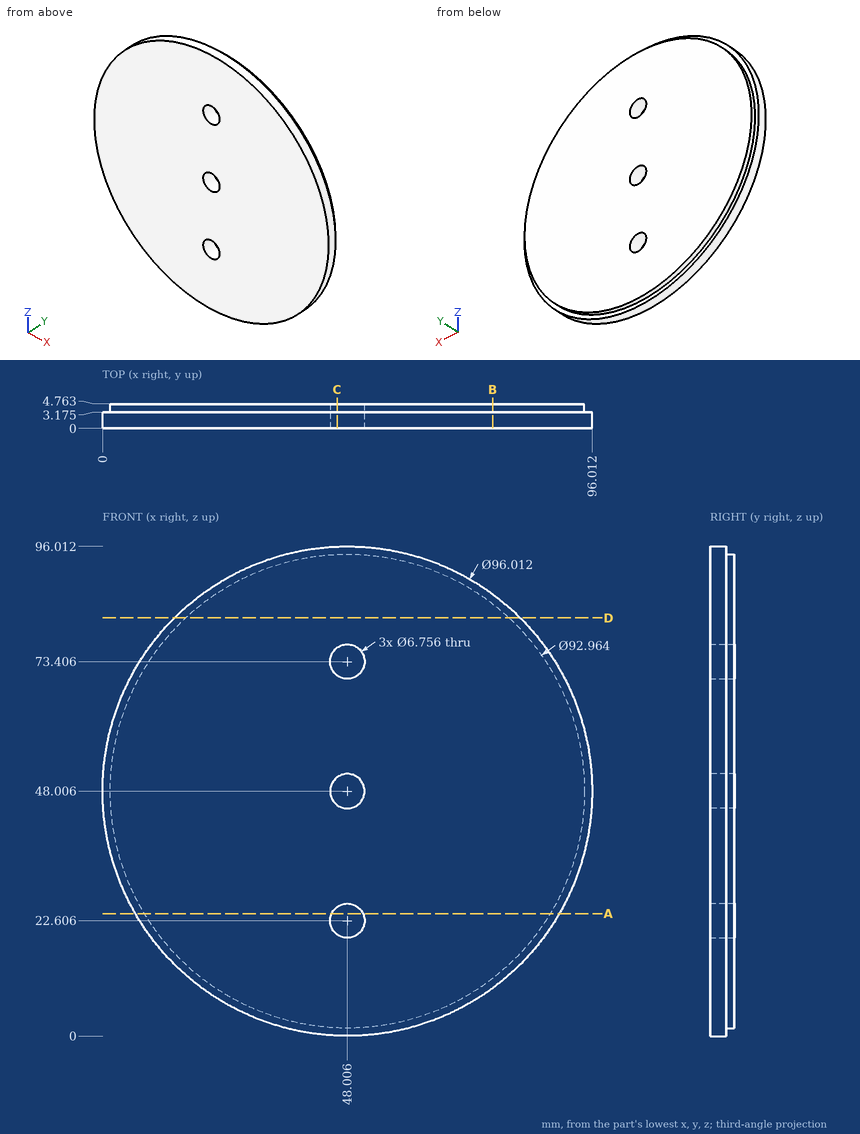
Geometry: see drawing. Coordinates: mm, zero at the bounding-box minimum. Round coordinates to 2 decimals unless told otherwise and drop trailing zeros. Loops run counter-clockwise (first coordinate to the right, second up) from the corner with the lowest first, then second, coordinate; pieces in that order, holes last. Notation, with made-up numbers: M -37.75,53 L -26.75,53 A24 ccw -26.75,77 Z; hole C 56.25,-5.75 d9. An arc over 180 degrees is marked long. Use a Markdown table: item, result. Add a question column.
1. Ray query, line 1 along Z through (x, y) = (48.5, 2.5) (1 decimal); line 2 along Z through (x, y) = (47, 2.85); line 3 along X through (y, z) = (1.9, 47.5) (1 decimal). Return the intervals inside material, ascending. Write a range as [from, to].
2. Cut plane D-D, the plane z = 82. Output: boundary loops of the cut face in (x, y) (1 decimal), and give its area (3 significant figures).
3. Cut plane A-A, the plane z = 24. Output: boundary loops of the cut face in (x, y) (1 decimal).
4. Cut plane C-C, the plane x = 46. Output: boundary loops of the cut face in (y, z) (1 decimal).
5. Contact query for a flat-ended pin moving along its axis: pin 1 (6 mm diameter, centred on x = 48.006, z = 73.406, fed in from -Y). Output: stop coordinate, or through.
6. Cut plane B-B, the plane x = 76.5. Output: boundary loops of the cut face in (y, z) (1 decimal), and give its area (3 significant figures).
Solution:
| question | item | result |
|---|---|---|
| 1 | line 1 | z = [0, 19.3], [25.9, 44.7], [51.3, 70.1], [76.7, 96] |
| 1 | line 2 | z = [0.01, 19.38], [25.83, 44.78], [51.23, 70.18], [76.63, 96] |
| 1 | line 3 | x = [0, 44.7], [51.3, 96] |
| 2 | outline | M 14.1,0 L 81.9,0 L 81.9,3.2 L 79.7,3.2 L 79.7,4.8 L 16.3,4.8 L 16.3,3.2 L 14.1,3.2 Z |
| 2 | area | 316 mm2 |
| 3 | outline | M 6.4,0 L 44.9,0 L 44.9,4.8 L 8.2,4.8 L 8.2,3.2 L 6.4,3.2 Z; M 51.1,0 L 89.6,0 L 89.6,3.2 L 87.8,3.2 L 87.8,4.8 L 51.1,4.8 Z |
| 4 | outline | M 0,0 L 3.2,0 L 3.2,1.6 L 4.8,1.6 L 4.8,19.9 L 0,19.9 Z; M 0,25.3 L 4.8,25.3 L 4.8,45.3 L 0,45.3 Z; M 0,50.7 L 4.8,50.7 L 4.8,70.7 L 0,70.7 Z; M 0,76.1 L 4.8,76.1 L 4.8,94.4 L 3.2,94.4 L 3.2,96 L 0,96 Z |
| 5 | pin 1 | passes through |
| 6 | outline | M 0,9.4 L 3.2,9.4 L 3.2,11.3 L 4.8,11.3 L 4.8,84.7 L 3.2,84.7 L 3.2,86.6 L 0,86.6 Z |
| 6 | area | 362 mm2 |
